CAD build for the part. Positions are in the model's coordinates, mm. A direction names the side the tool comes from. Round coordinates to 2 decimals unless told otherwise and drop trailing zeros. Loops run counter-clockwise (first coordinate to the right, second up) from the corner with the lowest first, then second, coordinate; pieces in that order, holes last. Notation, with made-up numbers: M 44.25,41 L 76.25,41 A21 ccw 76.25,69 Z; hole C -11,-1 d10. An arc over 180 degrees is marked long. One line per item, written item: value. Start each with the question number.
Autodesk Inventor part; units mm, degrees
ref_plane "YZ Plane" through (0, 0, 0) normal (1, 0, 0) x (0, 1, 0)
ref_plane "XZ Plane" through (0, 0, 0) normal (0, 1, 0) x (-1, 0, 0)
ref_plane "XY Plane" through (0, 0, 0) normal (0, 0, 1) x (1, 0, 0)
sketch "Sketch1" plane through (0, 0, 0) normal (0, 1, 0) x (-1, 0, 0)
  circle A0 centre (0, 0) radius 12.7
  circle A1 centre (0, 0) radius 25.4
  line L0 (-12.7, -21.997) -> (-95.25, -21.997)
  line L1 (-95.25, 21.997) -> (-12.7, 21.997)
  arc A2 (-63.5, -9.525) -> (-63.5, 9.525) centre (-63.5, 0) ccw
  line L2 (-63.5, 9.525) -> (-95.25, 9.525)
  line L3 (-78.5703, 0) -> (-63.5, 0) construction
  line L4 (-63.5, -9.525) -> (-95.25, -9.525)
  line L5 (-95.25, -21.997) -> (-95.25, -9.525)
  line L6 (-95.25, 9.525) -> (-95.25, 21.997)
  line L7 (-44.45, 21.997) -> (-44.45, 12.472)
  line L8 (-44.45, 12.472) -> (-22.1271, 12.472)
  line L9 (-52.07, 21.997) -> (-52.07, -21.997)
  dimension "d0" = 25.4
  dimension "d3" = 19.05
  dimension "d4" = 31.75
  dimension "d5" = 12.7
  dimension "d6" = 44.45
  dimension "d7" = 9.525
  dimension "d8" = 7.62
  dimension "d9" = 82.55
  dimension "d10" = 12.7
extrude "Extrusion3" add sketch "Sketch1" along normal blind 50.8 contours A1
extrude "Extrusion4" add sketch "Sketch1" along normal blind 6.35 contours A1 L8 L7 L1 | L0 L9 L1 L7 L8 A1 | L0 L5 L4 A2 L2 L6 L1 L9
properties part number "Distance from Face"
(1) Slice it at C-C, the plane y = 47. List the corners of the cut face in (x, z).
(2) Probe L1, parallel to Z at x = 0, y = 17; L2, parallel to Y at x = 48, z = 10; L3, parallel to Z at x = -4.5, y = 11.5. List the from-to ranges inside material, lowest first.
(3) Slice it at A-A, the plane z = 0. List the corners of the cut face in (x, y) (3 decimals).
(4) Slice it at B-B, the plane x = 0. List the corners of the cut face in (y, z).
(5) Flat gauge pins, fed straight in: P1, Ø6, axis at x = 30.5, z = -19.5, coming from the +Y side; P2, Ø3, axis at x = 68, y = 2.5, coming from the +Z side; P3, Ø4, axis at x = -0.5, z = 10, coming from the -Y side; P4, Ø6, axis at y = 11, z = 7.5, coming from the -X side. Where does each tip first touch, or does it go through?
(6) Which spindle directions (+Z, -Z, +X, -X, +Y, -Y) get a long thin tool onto all of the face, cutting with end or side? Do faces 1 (the flat face through (53, 3, -21.997)), 2 (the flat face through (79, 3, 9.525)), 3 (the flat face through (36, 0, 0)), 4 (the flat face through (55, 3, 21.997)). Say none if no direction does.
(7) Slice it at D-D, the plane x = 39.5. List the corners of the cut face in (y, z), and give its area (3 significant figures).
(8) Mould opens along Z. For faces 5 (the flat face through (79, 3, -9.525)), 6 (the cylindrical face through (-24.227, 25.044, -7.629)), 7 (the flat face through (55, 6.35, 5)) say: pulls with the +Z half, pulls with the -Z half, needs draft (parallel to the pull), parting line crosses it, or undercut.
Check result:
1. outline: C 0,0 d50.8; hole C 0,0 d25.4
2. L1: z = -25.4 to -12.7, 12.7 to 25.4
2. L2: y = 0 to 6.35
2. L3: z = -25 to -11.88, 11.88 to 25
3. outline: M -25.4,0 L -12.7,0 L -12.7,50.8 L -25.4,50.8 Z; M 12.7,0 L 53.975,0 L 53.975,6.35 L 25.4,6.35 L 25.4,50.8 L 12.7,50.8 Z
4. outline: M 0,-25.4 L 50.8,-25.4 L 50.8,-12.7 L 0,-12.7 Z; M 0,12.7 L 50.8,12.7 L 50.8,25.4 L 0,25.4 Z
5. P1: stops at y = 6.35
5. P2: stops at z = 22
5. P3: passes through
5. P4: stops at x = -25
6. face 1: -Z, +X, +Y, -Y
6. face 2: +X, +Y, -Y
6. face 3: +Z, -Z, +X, -X, -Y
6. face 4: +Z, +X, +Y, -Y
7. outline: M 0,-22 L 6.35,-22 L 6.35,22 L 0,22 Z
7. area: 279 mm^2
8. face 5: undercut
8. face 6: parting line crosses it
8. face 7: needs draft
